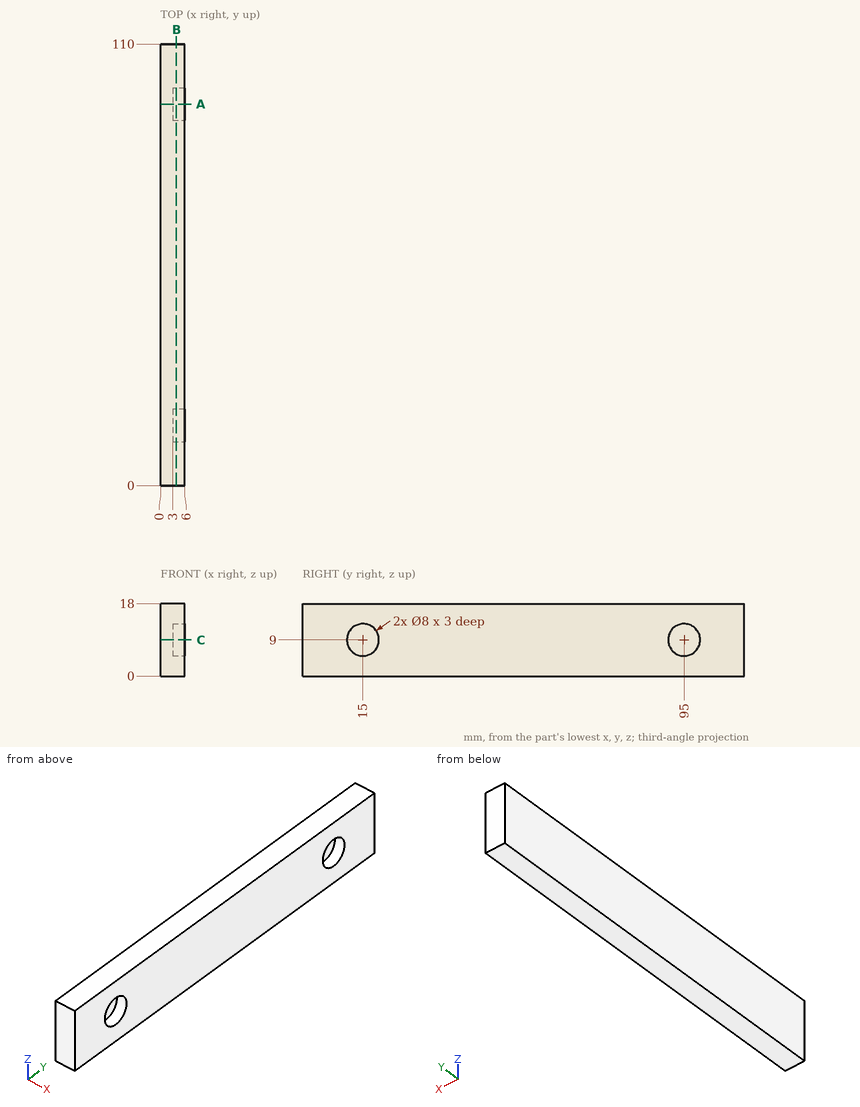
Can you work these out from the drawing? Everything is in mm from the part's minimum corner. Coordinates: 2 decimals unless noted, no trailing zeros. Write each loop counter-clockwise with the first axis right and the second up, starting at its lowest first coordinate (ties: lowest second). Pieces come first, ordered by that corner, then holes. Notation, with made-up numbers: (60, 53) -> (89, 53) arc R14 ccw to (89, 73) -> close; hole circle Ø6 at (-11.5, 46). An arc over 180 degrees is marked (long way). Write item = value, one per line.
(1) Imagine slicing it at A-A (y = 95). Please give me the cut outline in (x, z), and give its area (3 significant figures).
Verdict:
outline = (0, 0) -> (6, 0) -> (6, 5) -> (3, 5) -> (3, 13) -> (6, 13) -> (6, 18) -> (0, 18) -> close
area = 84.0 mm^2
(2) Imagine slicing it at B-B (x = 3.95). Please give me the cut outline in (y, z).
Verdict:
outline = (0, 0) -> (110, 0) -> (110, 18) -> (0, 18) -> close; hole circle Ø8 at (15, 9); hole circle Ø8 at (95, 9)
(3) Imagine slicing it at C-C (z = 9). Please give me the cut outline in (x, y), and give its area (3 significant figures).
Verdict:
outline = (0, 0) -> (6, 0) -> (6, 11) -> (3, 11) -> (3, 19) -> (6, 19) -> (6, 91) -> (3, 91) -> (3, 99) -> (6, 99) -> (6, 110) -> (0, 110) -> close
area = 612 mm^2
(4) If I drill on probe 1 along Z at (x, y) = (3.6, 15); probe 2 along Y at (x, z) = (5.1, 8.5); probe 3 along Z at (x, y) = (5.75, 16.5), over which ranges is the centre line in solid material (lowest first)?
Verdict:
probe_1 = 0 to 5, 13 to 18
probe_2 = 0 to 11.03, 18.97 to 91.03, 98.97 to 110
probe_3 = 0 to 5.29, 12.71 to 18
(5) For pin 1 (2 mm diameter, centred on x = 1, z = 11, fed in from -Y); pin 2 (4 mm diameter, centred on y = 15, z = 7.5, fed in from +X), each with a flat end and sliding along its axis, tell me the tip position at first contact or that it passes through.
Verdict:
pin_1 = 0
pin_2 = 3
